from build123d import *

# Parameters (mm, degrees)
F1_DEPTH = 13
F2_W     = 132.4155251533
F2_H     = 17.2680690885
F3_DEPTH = 13
F4_W     = 100.1826098412
F4_H     = 29.5549705625
F5_DEPTH = 13
F6_W     = 122.0997741669
F6_H     = 33.8719934225
F7_DEPTH = 13


# Not quite as in the source:
# - the program builds the solid bodies; features that only make, move or delete a surface that nothing else refers to are left out


with BuildPart() as f1:
    # F0 (on Front) → F1 (new body)
    with BuildSketch(Plane.XZ):
        with BuildLine():
            Line((144.5844748467, 101.5557457248), (-79.4445127249, 101.5557457248))
            Line((-79.4445127249, 101.5557457248), (-79.4445127249, 57.1600347757))
            Line((-79.4445127249, 57.1600347757), (-132.4155251533, 57.1600347757))
            Line((-132.4155251533, 57.1600347757), (-132.4155251533, -108.4442542752))
            Line((-132.4155251533, -108.4442542752), (164.5844748467, -108.4442542752))
            Line((164.5844748467, -108.4442542752), (164.5844748467, 81.5557457248))
            ThreePointArc((164.5844748467, 81.5557457248), (158.7266104705, 95.6978813486), (144.5844748467, 101.5557457248))
        make_face()
    extrude(amount=F1_DEPTH)

    # F2 (on face) → F3 (cut)
    with BuildSketch(Plane.XZ.offset(13)):
        with Locations((-66.2077625766, -85.9657116234)):
            Rectangle(F2_W, F2_H)
    extrude(amount=-F3_DEPTH, mode=Mode.SUBTRACT)

    # F4 (on face) → F5 (cut)
    with BuildSketch(Plane.XZ.offset(13)):
        with Locations((114.4931699261, 51.3486675918)):
            Rectangle(F4_W, F4_H)
    extrude(amount=-F5_DEPTH, mode=Mode.SUBTRACT)

    # F6 (on face) → F7 (cut)
    with BuildSketch(Plane.XZ.offset(13)):
        with Locations((103.5345877632, -66.7051747441)):
            Rectangle(F6_W, F6_H)
    extrude(amount=-F7_DEPTH, mode=Mode.SUBTRACT)


solid = f1.part
Verification items for the finished model (mm, model axes). A direction names the side the tool comes from. Round coordinates to 2 decimals unless told otherwise and drop trailing zeros. Loops run counter-clockwise (first coordinate to the right, second up) from the corner with the lowest first, then second, coordinate; pieces in that order, holes last. Notation, with made-up numbers: (-7.75, 84.25) - (12.25, 84.25) arc R25 ccw to (12.25, 120.25) - close; hole circle Ø3 at (1, -20). An arc over 180 degrees is marked (long way). Use one line per item in the form item = value.
1. Draft check along Z on faces 1 (the flat face through (34, -6, 101.556)), 2 (the flat face through (14, -13, -2)), 3 (the flat face through (64.402, -7, 51)), 4 (the flat face through (14, -6, -108.444)). Enter one of: pulls with the +Z half, pulls with the -Z half, needs draft (parallel to the pull), parting line crosses it, or undercut.
A:
face_1 = pulls with the +Z half
face_2 = needs draft
face_3 = undercut
face_4 = pulls with the -Z half
2. Section check C-C on y = -3.25. Record the cut outline in (x, z).
A:
outline = (-132.42, -108.44) - (164.58, -108.44) - (164.58, -83.64) - (42.48, -83.64) - (42.48, -49.77) - (164.58, -49.77) - (164.58, 36.57) - (64.4, 36.57) - (64.4, 66.13) - (164.58, 66.13) - (164.58, 81.56) arc R20 ccw to (144.58, 101.56) - (-79.44, 101.56) - (-79.44, 57.16) - (-132.42, 57.16) - (-132.42, -77.33) - (0, -77.33) - (0, -94.6) - (-132.42, -94.6) - close
3. Section check B-B on x = -53.5. Record the cut outline in (y, z).
A:
outline = (-13, -108.44) - (0, -108.44) - (0, -94.6) - (-13, -94.6) - close; (-13, -77.33) - (0, -77.33) - (0, 101.56) - (-13, 101.56) - close
4. Access from +Z, -Z, +X, -X, +Y, -Y to the whole of each face (thin tool, end or side, straight path). Record for faces 5 (the flat face through (103, -7, -83.641)), 6 (the flat face through (-67, -7, -94.6)), 7 (the flat face through (-132.416, -6, -101)), 8 (the flat face through (-79.445, -6, 80)).
A:
face_5 = +X, +Y, -Y
face_6 = -X, +Y, -Y
face_7 = +Z, -Z, -X, +Y, -Y
face_8 = +Z, -X, +Y, -Y
5. Section check D-D on z = -54. Record the cut outline in (x, y).
A:
outline = (-132.42, -13) - (42.48, -13) - (42.48, 0) - (-132.42, 0) - close
6. Scan lines: probe 1 along Z at (x, y) = (72, -9.25); probe 2 along Z at (x, y) = (-62.5, -12); probe 3 along Z at (x, y) = (46.5, -5). Record each from-to range of solid material in increasing order.
A:
probe_1 = -108.44 to -83.64, -49.77 to 36.57, 66.13 to 101.56
probe_2 = -108.44 to -94.6, -77.33 to 101.56
probe_3 = -108.44 to -83.64, -49.77 to 101.56
7. Section check A-A on x = 125. Record the cut outline in (y, z).
A:
outline = (-13, -108.44) - (0, -108.44) - (0, -83.64) - (-13, -83.64) - close; (-13, -49.77) - (0, -49.77) - (0, 36.57) - (-13, 36.57) - close; (-13, 66.13) - (0, 66.13) - (0, 101.56) - (-13, 101.56) - close
8. Gauge pin test, flat ends, axial feed: pin 1 Ø4 at (x, y) = (-106, -8.5) entering from +Z; pin 2 Ø6.5 at (y, z) = (-7, -72.5) entering from +X. Record the tip position at first contact, or that the pin passes through.
A:
pin_1 = 57.16
pin_2 = 42.48
